Can you work these out from the model? Positions are in its coordinate system, mm. Face numbers are marked on the shaded views. Round coordinates to 2 decimals unless told otherwise and drop trailing zeros. Write each loop counter-clockwise with the first axis right and the second up, starting at its lowest first coordinate (ties: lowest second). Pieces come first, ordered by that corner, then holes. Notation, with made-up numbers: M 34.25,68 L 84.25,68 A20 cw 84.25,99 Z; hole C 38,7 d7. An arc over 180 degrees is marked long. Answer in a Markdown table with one row per item. Add a question column.
(1) If I drill on probe 1 along Z at (x, y) = (1.5, 8.5); probe 2 along Z at (x, y) = (7.5, -8); probe 3 along Y at (x, z) = (5.25, 7), over which ranges is the centre line in solid material (lowest first)?
(2) Suppose I cut it at A-A, the plane z = 0. Write out the boundary of the cut face in (x, y).
(3) If we mould it in two halves opening along Y, with no side actions, what happens to the marked faces 1, 2 and 3? For each: released by +Y, released by -Y, zero draft, split by the parting line, or undercut.
(4) Suppose I cut it at C-C, the plane x = 2.25. Write out the boundary of the cut face in (y, z).
(5) Suppose I cut it at D-D, the plane z = 8. Count the separate pieces of the cut face and the enclosed holes in it, then the cut area to 3 significant figures.
(6) I'm going to push flat-ended pins straight in: pin 1 (4 mm diameter, centred on x = 1, y = 22.5, fed in from +Z); pin 2 (5 mm diameter, centred on y = 11, z = -17.5, fed in from -X); pin 3 (5 mm diameter, centred on x = 3, y = -20, fed in from -Z); pin 4 (4 mm diameter, centred on x = 7.5, y = -11.5, fed in from -Z). Where does each tip first touch, or does it pass through?
Autodesk Inventor part; units mm, degrees
ref_plane "YZ Plane" through (0, 0, 0) normal (1, 0, 0) x (0, 1, 0)
ref_plane "XZ Plane" through (0, 0, 0) normal (0, 1, 0) x (-1, 0, 0)
ref_plane "XY Plane" through (0, 0, 0) normal (0, 0, 1) x (1, 0, 0)
sketch "Sketch1" plane through (0, 0, 0) normal (1, 0, 0) x (0, 1, 0)
  circle A0 centre (0, 0) radius 29
  circle A1 centre (0, 0) radius 22.2155 construction
  circle A2 centre (0, 0) radius 29
  dimension "d21" = 58
  dimension "d28" = 58
extrude "Extrusion1" add sketch "Sketch1" along normal blind 10
sketch "Sketch2" plane through (0, 0, 0) normal (-1, 0, 0) x (0, 0, 1)
  point P0 (0, 0)
  point P1 (8, 8)
  point P2 (8, -8)
  point P3 (-8, -8)
  point P4 (-8, 8)
  dimension "d2" = 8
  dimension "d3" = 8
  dimension "d4" = 16
  dimension "d5" = 16
hole "Hole1" at (0, 8, 8) at (0, -8, 8) at (0, -8, -8) at (0, 8, -8) direction (1, 0, 0) diameter 5 end through all
sketch "Sketch3" plane through (0, 0, 0) normal (-1, 0, 0) x (0, 0, 1)
  point P0 (0, 0)
  point P1 (0, 0)
hole "Hole2" at (0, 0, 0) direction (1, 0, 0) diameter 8 end through all
chamfer "Chamfer2" distance 1 distance2 1 1 edges at (10, -29, 0) measured on face at (10, -16.3716, 0)
equation "\"d21\" = d28"
properties part number "Tapon 2"
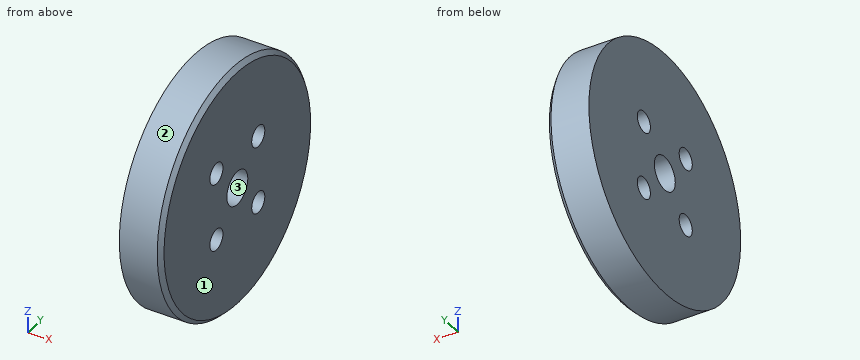
Calculated:
| question | item | result |
|---|---|---|
| 1 | probe 1 | -27.73 to -10.45, -5.55 to 5.55, 10.45 to 27.73 |
| 1 | probe 2 | -27.87 to -10.5, -5.5 to 5.5, 10.5 to 27.87 |
| 1 | probe 3 | -28.14 to -10.29, -5.71 to 5.71, 10.29 to 28.14 |
| 2 | outline | M 0,-29 L 9,-29 L 10,-28 L 10,-4 L 0,-4 Z; M 0,4 L 10,4 L 10,28 L 9,29 L 0,29 Z |
| 3 | face 1 | zero draft |
| 3 | face 2 | split by the parting line |
| 3 | face 3 | undercut |
| 4 | outline | C 0,0 d58; hole C -8,-8 d5; hole C -8,8 d5; hole C 0,0 d8; hole C 8,-8 d5; hole C 8,8 d5 |
| 5 | separate pieces | 3 |
| 5 | enclosed holes | 0 |
| 5 | area | 456 mm² |
| 6 | pin 1 | z = 20.51 |
| 6 | pin 2 | x = 0 |
| 6 | pin 3 | z = -23.12 |
| 6 | pin 4 | z = -27.4 |
